Autodesk Fusion 360 part; units mm, degrees
sketch "Sketch1" plane through (0, 0, 0) normal (0, 0, 1) x (1, 0, 0)
  line L0 (0, 0) -> (40.3, 0)
  line L1 (40.3, 0) -> (40.3, 128.54)
  line L2 (40.3, 128.54) -> (0, 128.54)
  line L3 (0, 128.54) -> (0, 0)
  line L4 (0, 0) -> (0, 3) construction
  line L5 (0, 3) -> (40.3, 3) construction
  line L6 (0, 0) -> (0, 17.3) construction
  line L7 (0, 17.3) -> (40.3, 17.3) construction
  line L8 (0, 17.3) -> (0, 30.3) construction
  line L9 (0, 30.3) -> (0, 47.6) construction
  line L10 (0, 47.6) -> (40.3, 47.6) construction
  line L11 (0, 30.3) -> (40.3, 30.3) construction
  line L12 (0, 47.6) -> (0, 78.9) construction
  line L13 (0, 78.9) -> (40.3, 78.9) construction
  line L14 (0, 78.9) -> (0, 99.2) construction
  line L15 (0, 99.2) -> (40.3, 99.2) construction
  line L16 (0, 128.54) -> (0, 110.04) construction
  line L17 (0, 110.04) -> (40.3, 110.04) construction
  line L18 (0, 0) -> (7, 0) construction
  line L19 (7, 0) -> (7, 47.6) construction
  line L20 (7, 0) -> (20, 0) construction
  line L21 (20, 0) -> (20, 47.6) construction
  line L22 (20, 0) -> (33, 0) construction
  line L23 (33, 0) -> (33, 47.6) construction
  circle A0 centre (7, 30.3) radius 3
  circle A1 centre (7, 17.3) radius 3
  circle A2 centre (20.15, 30.3) radius 3
  circle A3 centre (20.15, 17.3) radius 3
  circle A4 centre (33, 30.3) radius 3
  circle A5 centre (33, 17.3) radius 3
  circle A6 centre (7, 47.6) radius 3.3
  circle A7 centre (20, 47.6) radius 3.3
  circle A8 centre (33, 47.6) radius 3.3
  line L24 (0, 78.9) -> (20.15, 78.9) construction
  circle A9 centre (20.15, 78.9) radius 3.8
  line L25 (0, 99.2) -> (20.15, 99.2) construction
  circle A10 centre (20.15, 99.2) radius 2.5
  line L26 (0, 110.04) -> (0.6568, 110.04) construction
  line L27 (0, 110.04) -> (8.6, 110.04) construction
  line L28 (8.6, 110.04) -> (33.1, 110.04) construction
  circle A11 centre (8.6, 110.04) radius 3.8
  circle A12 centre (33.1, 110.04) radius 4.65
  line L29 (0, 3) -> (5, 3) construction
  line L30 (5, 3) -> (5, 4.5) construction
  line L31 (5, 3) -> (5, 1.5) construction
  line L32 (5, 1.5) -> (7.225, 1.5)
  line L33 (5, 1.5) -> (2.775, 1.5)
  line L34 (5, 4.5) -> (7.225, 4.5)
  line L35 (5, 4.5) -> (2.775, 4.5)
  line L36 (2.775, 3) -> (1.275, 3)
  arc A13 (2.775, 4.5) -> (2.775, 1.5) centre (2.775, 3) ccw
  line L37 (7.225, 3) -> (8.725, 3)
  arc A14 (7.225, 1.5) -> (7.225, 4.5) centre (7.225, 3) ccw
  arc A15 (2.775, 4.5) -> (2.775, 1.5) centre (2.775, 3) ccw
  line L38 (5, 4.5) -> (2.775, 4.5)
  line L39 (5, 4.5) -> (7.225, 4.5)
  arc A16 (7.225, 1.5) -> (7.225, 4.5) centre (7.225, 3) ccw
  line L40 (5, 1.5) -> (7.225, 1.5)
  line L41 (5, 1.5) -> (2.775, 1.5)
  line L42 (40.3, 0) -> (35.3, 0) construction
  line L43 (35.3, 0) -> (35.3, 3) construction
  arc A17 (33.075, 4.5) -> (33.075, 1.5) centre (33.075, 3) ccw
  line L44 (35.3, 4.5) -> (33.075, 4.5)
  line L45 (35.3, 4.5) -> (37.525, 4.5)
  line L46 (35.3, 1.5) -> (33.075, 1.5)
  line L47 (35.3, 1.5) -> (37.525, 1.5)
  arc A18 (37.525, 1.5) -> (37.525, 4.5) centre (37.525, 3) ccw
  line L48 (0, 128.54) -> (0, 125.74) construction
  line L49 (0, 125.74) -> (40.3, 125.74) construction
  line L50 (0, 125.74) -> (5, 125.74) construction
  line L51 (40.3, 125.74) -> (35.3, 125.74) construction
  arc A19 (2.775, 127.24) -> (2.775, 124.24) centre (2.775, 125.74) ccw
  line L52 (5, 127.24) -> (2.775, 127.24)
  line L53 (5, 127.24) -> (7.225, 127.24)
  line L54 (5, 124.24) -> (2.775, 124.24)
  line L55 (5, 124.24) -> (7.225, 124.24)
  arc A20 (7.225, 124.24) -> (7.225, 127.24) centre (7.225, 125.74) ccw
  arc A21 (33.075, 127.24) -> (33.075, 124.24) centre (33.075, 125.74) ccw
  line L56 (35.3, 127.24) -> (33.075, 127.24)
  line L57 (35.3, 127.24) -> (37.525, 127.24)
  line L58 (35.3, 124.24) -> (33.075, 124.24)
  line L59 (35.3, 124.24) -> (37.525, 124.24)
  arc A22 (37.525, 124.24) -> (37.525, 127.24) centre (37.525, 125.74) ccw
  dimension "d1" = 40.3
  dimension "d2" = 128.54
  dimension "d3" = 3
  dimension "d5" = 17.3
  dimension "d6" = 13
  dimension "d7" = 17.3
  dimension "d8" = 31.3
  dimension "d9" = 20.3
  dimension "d10" = 18.5
  dimension "d11" = 7
  dimension "d12" = 13
  dimension "d13" = 13
  dimension "d14" = 6
  dimension "d15" = 6
  dimension "d16" = 6
  dimension "d17" = 6
  dimension "d18" = 6
  dimension "d19" = 6
  dimension "d20" = 6.6
  dimension "d21" = 6.6
  dimension "d22" = 6.6
  dimension "d23" = 7.6
  dimension "d24" = 5
  dimension "d25" = 8.6
  dimension "d26" = 24.5
  dimension "d27" = 7.6
  dimension "d28" = 9.3
  dimension "d29" = 5
  dimension "d30" = 1.5
  dimension "d31" = 1.5
  dimension "d32" = 2.225
  dimension "d33" = 2.225
  dimension "d35" = 2.225
  dimension "d36" = 2.225
  dimension "d37" = 1.5
  dimension "d38" = 1.5
  dimension "d39" = 2.225
  dimension "d40" = 2.225
  dimension "d41" = 2.225
  dimension "d42" = 2.225
  dimension "d43" = 5
  dimension "d44" = 2.225
  dimension "d45" = 2.225
  dimension "d46" = 2.225
  dimension "d47" = 2.225
  dimension "d48" = 2.225
  dimension "d49" = 2.8
  dimension "d50" = 5
  dimension "d51" = 5
  dimension "d52" = 2.225
  dimension "d53" = 2.225
  dimension "d54" = 2.225
  dimension "d56" = 2.225
  dimension "d57" = 2.225
  dimension "d58" = 2.225
  dimension "d59" = 2.225
  dimension "d61" = 2.225
extrude "Extrude1" add sketch "Sketch1" along normal blind 2
equation "d32 = ( 4.45 / 2 ) * 1 mm"
equation "d33 = ( 4.45 / 2 ) * 1 mm"
equation "d35 = ( 4.45 / 2 ) * 1 mm"
equation "d36 = ( 4.45 / 2 ) * 1 mm"
equation "d39 = ( 4.45 / 2 ) * 1 mm"
equation "d40 = ( 4.45 / 2 ) * 1 mm"
equation "d41 = ( 4.45 / 2 ) * 1 mm"
equation "d42 = ( 4.45 / 2 ) * 1 mm"
equation "d44 = ( 4.45 / 2 ) * 1 mm"
equation "d45 = ( 4.45 / 2 ) * 1 mm"
equation "d46 = ( 4.45 / 2 ) * 1 mm"
equation "d47 = ( 4.45 / 2 ) * 1 mm"
equation "d48 = ( 4.45 / 2 ) * 1 mm"
equation "d52 = ( 4.45 / 2 ) * 1 mm"
equation "d53 = ( 4.45 / 2 ) * 1 mm"
equation "d54 = ( 4.45 / 2 ) * 1 mm"
equation "d56 = ( 4.45 / 2 ) * 1 mm"
equation "d57 = ( 4.45 / 2 ) * 1 mm"
equation "d58 = ( 4.45 / 2 ) * 1 mm"
equation "d59 = ( 4.45 / 2 ) * 1 mm"
equation "d61 = ( 4.45 / 2 ) * 1 mm"
Can you work these out from the model? Positions are in its coordinate system, mm. Coordinates: 2 decimals unless noted, no trailing zeros. Write each loop counter-clockwise with the first axis right and the second up, starting at its lowest first coordinate (ties: lowest second). Pieces come first, ordered by that corner, then holes. Notation, with made-up numbers: (10.5, 6) -> (33.5, 6) arc R25 ccw to (33.5, 36) -> close; hole circle Ø6 at (36.5, -39). An arc over 180 degrees is marked (long way). Write each question's results on one line, items separated by ' | '. Start each with the question number.
Item 1: If we section it at D-D, the plane x = 6: Write out the boundary of the cut face in (y, z).
Item 2: If we section it at A-A, the plane y = 3: Write out the boundary of the cut face in (x, z) (3 decimals), and give its area (3 significant figures).
Item 3: Thinking about a two-plate mould opening in X: for faces 1 (the cylindrical face through (19.28, 50.82, 0.99)), 2 (the flat face through (20, 65, 0)), which applies, released by +X, released by -X, zero draft, split by the parting line, or undercut?
Item 4: I'm going to push a flat-ended pin straight in: P1, Ø6, axis at x = 20.15, y = 78.9, coming from the -Z side. Where does the tip first touch, or does it pass through?
Item 5: If we section it at B-B, the plane y = 78.9: Write out the boundary of the cut face in (x, z).
Item 6: Please list where these lines run through material, in increasing order: probe 1 along X at (y, z) = (31, 0.8); probe 2 along Y at (x, z) = (20.15, 0.65); probe 3 along Y at (x, z) = (19.5, 0.75).
Item 7: If we section it at C-C, the plane z = 1.5: Count the separate pieces of the cut face and the enclosed holes in it, and give its area (3 significant figures).
Answer block:
1) outline: (0, 0) -> (1.5, 0) -> (1.5, 2) -> (0, 2) -> close; (4.5, 0) -> (14.47, 0) -> (14.47, 2) -> (4.5, 2) -> close; (20.13, 0) -> (27.47, 0) -> (27.47, 2) -> (20.13, 2) -> close; (33.13, 0) -> (44.46, 0) -> (44.46, 2) -> (33.13, 2) -> close; (50.74, 0) -> (107.27, 0) -> (107.27, 2) -> (50.74, 2) -> close; (112.81, 0) -> (124.24, 0) -> (124.24, 2) -> (112.81, 2) -> close; (127.24, 0) -> (128.54, 0) -> (128.54, 2) -> (127.24, 2) -> close
2) outline: (0, 0) -> (1.275, 0) -> (1.275, 2) -> (0, 2) -> close; (8.725, 0) -> (31.575, 0) -> (31.575, 2) -> (8.725, 2) -> close; (39.025, 0) -> (40.3, 0) -> (40.3, 2) -> (39.025, 2) -> close | area: 50.8 mm²
3) face 1: undercut | face 2: zero draft
4) P1: through
5) outline: (0, 0) -> (16.35, 0) -> (16.35, 2) -> (0, 2) -> close; (23.95, 0) -> (40.3, 0) -> (40.3, 2) -> (23.95, 2) -> close
6) probe 1: 0 to 4.08, 9.92 to 17.23, 23.07 to 30.08, 35.92 to 40.3 | probe 2: 0 to 14.3, 20.3 to 27.3, 33.3 to 44.3, 50.9 to 75.1, 82.7 to 96.7, 101.7 to 128.54 | probe 3: 0 to 14.37, 20.23 to 27.37, 33.23 to 44.34, 50.86 to 75.16, 82.64 to 96.79, 101.61 to 128.54
7) separate pieces: 1 | enclosed holes: 17 | area: 4,650 mm²
